Read the model definition and answer for the solid it produces. Units are mm, in the model's axes. A direction names the side the tool comes from. Give positions to 0.01 mm unless a question says otherwise; leave off trailing zeros. Order: outer loops, then holes, each group sorted by start corner. A loop starts at its lowest first (then second) coordinate and runs counter-clockwise, first axis right, second up. Notation, with made-up numbers: (59.5, -24) -> (98.5, -24) arc R22 ccw to (98.5, -1) -> close; hole circle Ø3 at (65.25, 58.5). An arc over 180 degrees is marked (long way). Answer as CSV lines item,"result". Start each with the question number.
1) A flat-ended cylindrical pin translates along its axis: pin 1 Ø1 at (x, y) = (1.5, 0.5) entering from -Z. Find the tip coordinate at first contact, or state that the pin passes through.
2) Find section D-D (x = 0). Determine the outline of the cut face in (y, z), and give its area (3 significant figures).
3) Find section A-A (y = 1.05). Determine the outline of the cut face in (x, z), and give its area (3 significant figures).
4) Find section C-C (x = -2.5). Determine the outline of the cut face in (y, z).
5) The mould has two halves that part along X. Classify faces 1 (the face through (0, 1, 6)), 2 (the face through (1.6, 1, -2.8)), 3 (the face through (1, 0, 3)): +X half, -X half, draft (parallel to the pull), parting line (faces both ways), or undercut.
6) Find section B-B (z = 1). Determine the outline of the cut face in (x, y).
7) Straight lines are drawn through the part: L1, parallel to X at y = 1.25, z = 1.75; L2, parallel to Z at x = 2.5, y = 1; L3, parallel to Z at x = 0, y = 0.15. For each, find the intervals that lie inside material, in ascending order. Write a range as from..to.
8) For faces 4 (the face through (-1.6, 0.99, -2.81)), 5 (the face through (-2.404, 0.986, -4.738)), determine the directions among +Z, -Z, +X, -X, +Y, -Y from which every point of the face is accessible in a straight line to the end or side of a thin tool.
```python
from build123d import *

# Parameters (mm, degrees)
BOSS_EXTRUDE1_DEPTH = 2


with BuildPart() as part:
    # Sketch1 → Boss-Extrude1 (new body)
    with BuildSketch(Plane(origin=(0, 0, 0), x_dir=(1, 0, 0), z_dir=(0, 1, 0))):
        with BuildLine():
            ThreePointArc((3, 0), (0, -3), (-3, 0))
            ThreePointArc((-3, 0), (-2.743755194, 1.213180711), (-2.018795042, 2.219113918))
            ThreePointArc((-2.018795042, 2.219113918), (-1.982332969, 2.251745101), (-1.945343535, 2.283777251))
            ThreePointArc((-1.945343535, 2.283777251), (-1.596748035, 2.82076449), (-1.5319755, 3.457693556))
            ThreePointArc((-1.5319755, 3.457693556), (-2.424767696, 4.747181988), (-3.972947107, 4.496186305))
            ThreePointArc((-3.972947107, 4.496186305), (0, -6), (3.972947107, 4.496186305))
            ThreePointArc((3.972947107, 4.496186305), (2.424767696, 4.747181988), (1.5319755, 3.457693556))
            ThreePointArc((1.5319755, 3.457693556), (1.590995928, 2.827214748), (1.932969653, 2.294259864))
            ThreePointArc((1.932969653, 2.294259864), (1.976239555, 2.257094863), (2.018795042, 2.219113918))
            ThreePointArc((2.018795042, 2.219113918), (2.743755194, 1.213180711), (3, 0))
        make_face()
    extrude(amount=BOSS_EXTRUDE1_DEPTH)


solid = part.part
```
Findings below:
1,pin 1,"z = -4.47"
2,outline,"(0, 3) -> (2, 3) -> (2, 6) -> (0, 6) -> close"
2,area,"6.00 mm²"
3,outline,"(-3.97, -4.5) arc R1.47 ccw to (-1.53, -3.46) arc R1.36 ccw to (-1.95, -2.28) arc R3 cw to (-2.02, -2.22) arc R3 cw (long way) to (2.02, -2.22) arc R3 cw to (1.93, -2.29) arc R1.34 ccw to (1.53, -3.46) arc R1.47 ccw to (3.97, -4.5) arc R6 ccw (long way) to start"
3,area,"72.2 mm²"
4,outline,"(0, -4.78) -> (2, -4.78) -> (2, -1.66) -> (0, -1.66) -> close; (0, 1.66) -> (2, 1.66) -> (2, 5.45) -> (0, 5.45) -> close"
5,face 1,"parting line"
5,face 2,"undercut"
5,face 3,"draft"
6,outline,"(-5.92, 0) -> (-2.83, 0) -> (-2.83, 2) -> (-5.92, 2) -> close; (2.83, 0) -> (5.92, 0) -> (5.92, 2) -> (2.83, 2) -> close"
7,L1,"-5.74..-2.44, 2.44..5.74"
7,L2,"-4.78..-1.66, 1.66..5.45"
7,L3,"3..6"
8,face 4,"+Y, -Y"
8,face 5,"-Z, +Y, -Y"
